Source: three-view drawing plus pictorial views. Frame: mm from the lowest corner of the part. Round coordinates to 2 decimals unless told otherwise and drop trailing zeros. Loops run counter-clockwise (first coordinate to the right, second up) from the corner with the lowest first, then second, coordinate; pieces in that order, holes last. Notation, with made-up numbers: (83.25, 57) -> (121.25, 57) arc R23 ccw to (121.25, 77) -> close; hole circle Ø2 at (9.5, 15.25). An arc over 180 degrees is marked (long way). Answer in a Markdown table with one row per item. Add a question column.
Q1. Section A-A, the plane z = 1. Output: boundary loops of the cut face in (x, y) (1 decimal).
Q2. Section C-C, the plane y = 28. Output: boundary loops of the cut face in (x, z) (1 decimal).
Q3. Mould query, pull axis Y, two halves, no side actions, for the marked faces 1 and 2. Classes: pulls with the +Y half, pulls with the -Y half, needs draft (parallel to the pull), parting line crosses it, or undercut.
Q4. Ray query, L1, parallel to X at y = 28.5, z = 5.5; L2, parallel to Z at x = 20, y = 43.5; L3, parallel to X at y = 6, z = 7.5 (1 decimal). Return the intervals inside material, ascending. Write a range as from..to.
Q5. Pin query (flat end, axial travel): pin 1 (1.5 mm diameter, centred on x = 6, z = 1, fed in from -Y); pin 2 (2.5 mm diameter, centred on x = 68, y = 26.5, fed in from +Z); pin 3 (3.5 mm diameter, centred on x = 4, z = 1, fed in from +Y). Return the tip coordinate at first contact, or that it passes through.
Q6. Section B-B, the plane x = 4. Output: boundary loops of the cut face in (y, z).
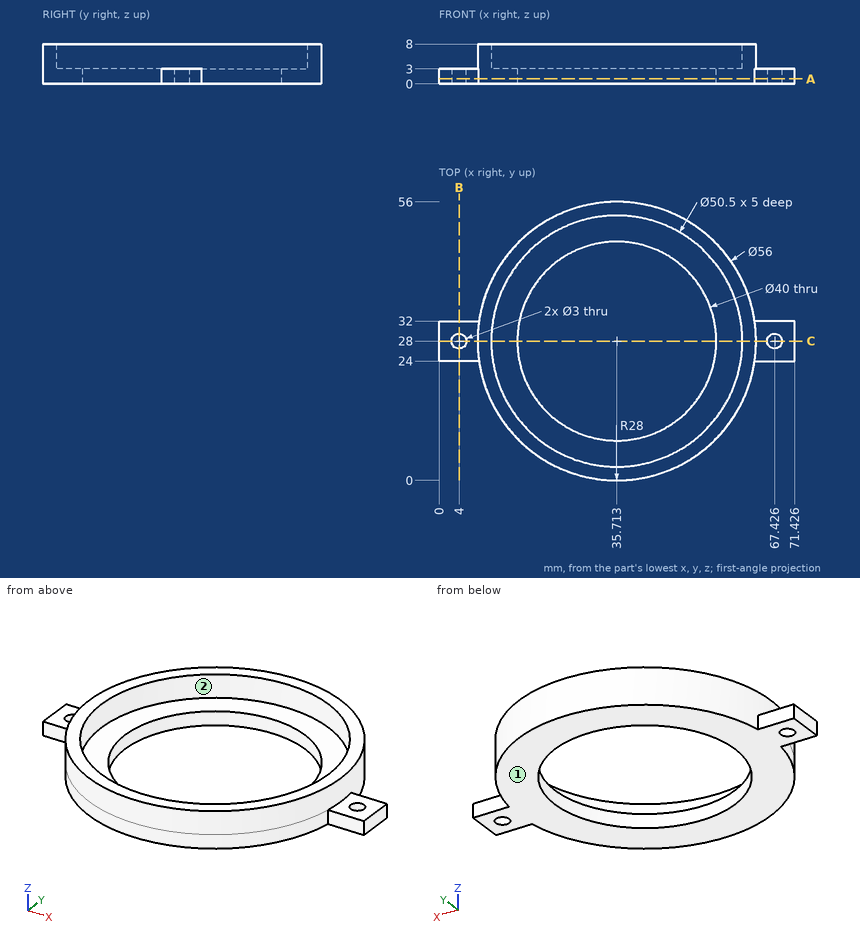
Answer block:
| question | item | result |
|---|---|---|
| 1 | outline | (0, 24) -> (8, 24) arc R28 ccw to (63.4, 24) -> (71.4, 24) -> (71.4, 32) -> (63.4, 32) arc R28 ccw to (8, 32) -> (0, 32) -> close; hole circle Ø3 at (4, 28); hole circle Ø40 at (35.7, 28); hole circle Ø3 at (67.4, 28) |
| 2 | outline | (0, 0) -> (2.5, 0) -> (2.5, 3) -> (0, 3) -> close; (5.5, 0) -> (15.7, 0) -> (15.7, 3) -> (10.5, 3) -> (10.5, 8) -> (7.7, 8) -> (7.7, 3) -> (5.5, 3) -> close; (55.7, 0) -> (65.9, 0) -> (65.9, 3) -> (63.7, 3) -> (63.7, 8) -> (61, 8) -> (61, 3) -> (55.7, 3) -> close; (68.9, 0) -> (71.4, 0) -> (71.4, 3) -> (68.9, 3) -> close |
| 3 | face 1 | needs draft |
| 3 | face 2 | undercut |
| 4 | L1 | 7.72..10.47, 60.96..63.71 |
| 4 | L2 | 0..3 |
| 4 | L3 | 18.4..23.3, 48.1..53 |
| 5 | pin 1 | y = 24 |
| 5 | pin 2 | z = 3 |
| 5 | pin 3 | y = 32 |
| 6 | outline | (24, 0) -> (26.5, 0) -> (26.5, 3) -> (24, 3) -> close; (29.5, 0) -> (32, 0) -> (32, 3) -> (29.5, 3) -> close |
